```python
from build123d import *

# Parameters (mm, degrees)
SKETCH_1_R          = 4
SKETCH_1_R_2        = 3.15
EXTRUDE_1_DEPTH     = 149
EXTRUDE_START       = 1
SKETCH_3_R          = 4
EXTRUDE_2_DEPTH     = 1
EXTRUDE_START_2     = -80
SKETCH_4_2_R        = 10.5
SKETCH_4_2_R_2      = 4
EXTRUDE_4_DEPTH     = 30
EXTRUDE_START_3     = -10
SKETCH_4_R          = 10.5
SKETCH_4_R_2        = 4
EXTRUDE_3_DEPTH     = 28
SKETCH_5_R          = 3.15
CUT_EXTRUDE_1_DEPTH = 10


with BuildPart() as part:
    # 草图1 → 凸台-拉伸1 (new body)
    with BuildSketch(Plane.XY):
        Circle(SKETCH_1_R)
        Circle(SKETCH_1_R_2, mode=Mode.SUBTRACT)
    extrude(amount=EXTRUDE_1_DEPTH)

    # 草图3 → 凸台-拉伸2 (add)
    with BuildSketch(Plane(origin=(0, 0, 0), x_dir=(-1, 0, 0), z_dir=(0, 0, -1)).offset(EXTRUDE_START)):
        Circle(SKETCH_3_R)
    extrude(amount=-EXTRUDE_2_DEPTH)

    # 草图4<2> → 凸台-拉伸4 (add)
    with BuildSketch(Plane(origin=(0, 0, -1), x_dir=(-1, 0, 0), z_dir=(0, 0, -1)).offset(EXTRUDE_START_2)):
        Circle(SKETCH_4_2_R)
        Circle(SKETCH_4_2_R_2, mode=Mode.SUBTRACT)
    extrude(amount=-EXTRUDE_4_DEPTH)

    # 草图4 → 凸台-拉伸3 (add)
    with BuildSketch(Plane(origin=(0, 0, -1), x_dir=(-1, 0, 0), z_dir=(0, 0, -1)).offset(EXTRUDE_START_3)):
        Circle(SKETCH_4_R)
        Circle(SKETCH_4_R_2, mode=Mode.SUBTRACT)
    extrude(amount=-EXTRUDE_3_DEPTH)

    # 草图5 → 切除-拉伸1 (cut)
    with BuildSketch(Plane(origin=(0, 0, -1), x_dir=(-1, 0, 0), z_dir=(0, 0, -1))):
        Circle(SKETCH_5_R)
    extrude(amount=-CUT_EXTRUDE_1_DEPTH, mode=Mode.SUBTRACT)


solid = part.part
```
Geometry check sheet. Reference: the model listing, model coordinates, mm. A direction names the side the tool comes from. Coordinates: 2 decimals unless noted, no trailing zeros. Order: outer loops, then holes, each group sorted by start corner. A loop starts at its lowest first (then second) coordinate and runs counter-clockwise, first axis right, second up.
Item 1: Mould release check, pull along Z, two halves, no side actions. Record for faces 1 (the cylindrical face through (-10, 3.2, 93.8)), 2 (the cylindrical face through (-0.867, -3.905, 57.706)), 3 (the flat face through (-2, -3, -1)): released by +Z, released by -Z, zero draft, split by the parting line, or undercut.
Item 2: Scan lines: line 1 along X through (y, z) = (0, 46.5); line 2 along Y through (x, z) = (0.25, 136); line 3 along Z through (x, y) = (4.75, -5.5). Record each from-to range of solid material in increasing order.
Item 3: Section check B-B (y = -9). Enter the section's corners in (x, z).
Item 4: Tool access check on faces 4 (the flat face through (-5, 0, 37)), 5 (the flat face through (-5, 0, 9)), 6 (the flat face through (-5, 0, 109)), 7 (the cylindrical face through (-10, 3.2, 22.8)). Record the directions out of +Z, -Z, +X, -X, +Y, -Y that give a thin tool (end or side, any length) a straight path to the whole face; none if there is none.
Item 5: Section check D-D (x = 8). Enter the section's corners in (y, z).
Item 6: Section check C-C (z = 68.5). Enter the section's corners in (x, y), plus the area to 3 significant figures.
Item 7: Depth check by flat-ended pin: pin 1 (1.5 mm diameter, centred on x = -3, z = 70.5, fed in from -Y); pin 2 (12 mm diameter, centred on x = -7, y = -8.5, fed in from -Z); pin 3 (1.5 mm diameter, centred on y = 5, z = 62.5, fed in from +X); pin 4 (6 mm diameter, centred on x = -3, z = 133.5, fed in from -Y). Enter the tip coordinate at first touch or a pass-through.
Item 8: Section check A-A (x = 0). Enter the section's corners in (y, z), plus the area to 3 significant figures.
Check sheet entries:
1. face 1: zero draft
1. face 2: undercut
1. face 3: released by -Z
2. line 1: x = -4 to -3.15, 3.15 to 4
2. line 2: y = -3.99 to -3.14, 3.14 to 3.99
2. line 3: z = 9 to 37, 79 to 109
3. outline: (-5.41, 9) - (5.41, 9) - (5.41, 37) - (-5.41, 37) - close; (-5.41, 79) - (5.41, 79) - (5.41, 109) - (-5.41, 109) - close
4. face 4: none
4. face 5: -Z
4. face 6: +Z
4. face 7: +Z, -Z
5. outline: (-6.8, 9) - (6.8, 9) - (6.8, 37) - (-6.8, 37) - close; (-6.8, 79) - (6.8, 79) - (6.8, 109) - (-6.8, 109) - close
6. outline: circle Ø8 at (0, 0); hole circle Ø6.3 at (0, 0)
6. area: 19.1 mm2
7. pin 1: stops at y = -3.31
7. pin 2: stops at z = 9
7. pin 3: passes through
7. pin 4: stops at y = -4
8. outline: (-10.5, 9) - (-4, 9) - (-4, -1) - (-3.15, -1) - (-3.15, 149) - (-4, 149) - (-4, 109) - (-10.5, 109) - (-10.5, 79) - (-4, 79) - (-4, 37) - (-10.5, 37) - close; (3.15, -1) - (4, -1) - (4, 9) - (10.5, 9) - (10.5, 37) - (4, 37) - (4, 79) - (10.5, 79) - (10.5, 109) - (4, 109) - (4, 149) - (3.15, 149) - close
8. area: 1,010 mm2
